```python
from build123d import *

# Parameters (mm, degrees)
F0_W     = 170
F0_H     = 330
F0_R     = 25
F0_R_2   = 10
F1_DEPTH = 40
F2_D     = 50
F4_DEPTH = 330.001


with BuildPart() as f1:
    # F0 (on Right) → F1 (new body)
    with BuildSketch(Plane.YZ):
        Rectangle(F0_W, F0_H)
        with Locations((0, -5)):
            Circle(F0_R, mode=Mode.SUBTRACT)
        with Locations((0, 125)):
            Circle(F0_R_2, mode=Mode.SUBTRACT)
        with Locations((0, -5)):
            Circle(F0_R)
    extrude(amount=-F1_DEPTH)

    # F2 (through all)
    with Locations(Plane.YZ):
        with Locations((0, -5)):
            Hole(F2_D / 2)

    # F3 (on face) → F4 (cut, through all)
    with BuildSketch(Plane(origin=(0, 0, -165), x_dir=(1, 0, 0), z_dir=(0, 0, -1))):
        with BuildLine():
            Line((0, -38.729833), (0, 38.729833))
            ThreePointArc((0, 38.729833), (-10, 0), (0, -38.729833))
        make_face()
    extrude(amount=-F4_DEPTH, mode=Mode.SUBTRACT)


solid = f1.part
```
CAD build for the part. Positions are in the model's coordinates, mm. Round coordinates to 2 decimals unless told otherwise and drop trailing zeros. Write each loop counter-clockwise with the first axis right and the second up, starting at its lowest first coordinate (ties: lowest second). Pieces come first, ordered by that corner, then holes. Notation, with made-up numbers: M 87,42 L 131,42 A25 ccw 131,77 Z; hole C -2.75,63 d2. An arc over 180 degrees is marked long. One line per question, with ' | ' between items.
1. Mould opens along Y. For faces 1 (the flat face through (0, -62, 2)), 2 (the flat face through (-20, 85, -2)), 3 (the cylindrical face through (-23.235, 24.976, -3.901)), 4 (the cylindrical face through (-24.47, 5.38, 133.43)) say: pulls with the +Y half, pulls with the -Y half, needs draft (parallel to the pull), parting line crosses it, or undercut.
Working result:
face 1: needs draft | face 2: pulls with the +Y half | face 3: undercut | face 4: undercut
2. Cut at B-B on z = -5. Write the cut outline in (x, y), and give its area (3 significant figures).
Working result:
outline: M -40,-85 L 0,-85 L 0,-38.73 A80 cw -5.99,-25 L -40,-25 Z; M -40,25 L -5.99,25 A80 cw 0,38.73 L 0,85 L -40,85 Z | area: 4,710 mm2
3. Cut at C-C on x = -29. Write the cut outline in (y, z).
Working result:
outline: M -85,-165 L 85,-165 L 85,165 L -85,165 Z; hole C 0,-5 d50; hole C 0,125 d20
4. Cut at D-D on z = 125. Write the cut outline in (x, y).
Working result:
outline: M -40,-85 L 0,-85 L 0,-38.73 A80 cw -9.37,-10 L -40,-10 Z; M -40,10 L -9.37,10 A80 cw 0,38.73 L 0,85 L -40,85 Z
5. Probe L1, parallel to Z at x = -31, y = 0; L2, parallel to Y at x = -25, z = 125; L3, parallel to Y at x = -31, z = -5. List the from-to ranges inside material, lowest first. Write a range as from..to.
Working result:
L1: -165..-30, 20..115, 135..165 | L2: -85..-10, 10..85 | L3: -85..-25, 25..85
6. Cut at A-A on y = 0. Write the cut outline in (x, z), and give its area (3 significant figures).
Working result:
outline: M -40,-165 L -10,-165 L -10,-30 L -40,-30 Z; M -40,20 L -10,20 L -10,115 L -40,115 Z; M -40,135 L -10,135 L -10,165 L -40,165 Z | area: 7,800 mm2
